Autodesk Inventor part; units mm, degrees
ref_plane "YZ Plane" through (0, 0, 0) normal (1, 0, 0) x (0, 1, 0)
ref_plane "XZ Plane" through (0, 0, 0) normal (0, 1, 0) x (-1, 0, 0)
ref_plane "XY Plane" through (0, 0, 0) normal (0, 0, 1) x (1, 0, 0)
ref_plane "РабПлоскость1" through (-185.8888, -38.5334, 331.0061) normal (0.9999756, 0.0023998, -0.0065586) x (-0.0066118, 0.0228778, -0.9997164)
sketch "Эскиз9" plane through (-185.8888, -38.5334, 331.0061) normal (0.9999756, 0.0023998, -0.0065586) x (-0.0066118, 0.0228778, -0.9997164)
  circle A0 centre (-0.0036, 0) radius 3.25
  line L0 (7.5744, -20.841) -> (-21.2183, 6.4584)
  line L1 (-21.2183, 6.4584) -> (-7.5816, 20.841)
  line L2 (-7.5816, 20.841) -> (21.2112, -6.4584)
  line L3 (21.2112, -6.4584) -> (7.5744, -20.841)
  line L4 (7.5744, -20.841) -> (-7.5816, 20.841) construction
  line L5 (-21.2183, 6.4584) -> (21.2112, -6.4584) construction
  line L6 (9.6794, 4.4753) -> (-3.9573, -9.9074)
  point P0 (330.5647, 30.5274)
extrude "Выдавливание4" add sketch "Эскиз9" along normal blind 6 contours L0 L1 L2 L6
fillet "Сопряжение2" radius 2 8 edges at (-182.8404, -48.5216, 334.7158) (-179.8019, -40.5311, 343.5115) (-185.8017, -40.5455, 343.5509) (-182.963, -33.8307, 321.4122) (-179.9244, -25.8402, 330.2079) (-185.9242, -25.8546, 330.2473) (-185.9016, -41.1833, 328.0837) (-179.9018, -41.1689, 328.0443)
sketch "Эскиз11" plane through (-185.7754, -31.0798, 351.0238) normal (0.0032506, 0.6712535, 0.7412207) x (0.9999756, 0.0023998, -0.0065586)
  line L0 (0, 17.8197) -> (6, -2)
  line L1 (6, 17.8197) -> (0, -2)
  line L2 (2.4, 11.0099) -> (3.6, 11.0099)
  line L3 (3.6, 11.0099) -> (3.6, 4.8099)
  line L4 (3.6, 4.8099) -> (2.4, 4.8099)
  line L5 (2.4, 4.8099) -> (2.4, 11.0099)
  line L6 (2.4, 11.0099) -> (3.6, 4.8099) construction
  line L7 (3.6, 11.0099) -> (2.4, 4.8099) construction
  point P0 (188.1477, 257.5062)
  point P1 (3, 7.9099)
  dimension "d31" = 1.2
  dimension "d32" = 6.2
extrude "Выдавливание6" cut sketch "Эскиз11" against normal blind 6
sketch "Эскиз12" plane through (-179.889, -38.519, 330.9668) normal (0.9999756, 0.0023998, -0.0065586) x (-0.0066118, 0.0228778, -0.9997164)
  line L0 (-16.5329, 11.4001) -> (-12.267, 15.8993)
  line L1 (-16.5329, 11.4001) -> (-12.1788, 7.2719)
  line L2 (-12.1788, 7.2719) -> (-7.913, 11.7711)
  line L3 (-12.267, 15.8993) -> (-7.913, 11.7711)
  line L4 (-12.1788, 7.2719) -> (-12.267, 15.8993)
  line L5 (-16.5329, 11.4001) -> (-7.913, 11.7711)
  circle A0 centre (-12.2229, 11.5856) radius 1.5
  point P0 (330.5647, 30.5274)
  dimension "d35" = 3
extrude "Выдавливание7" cut sketch "Эскиз12" against normal blind 6 contours A0 L4 L5 | L5 L4 A0 | A0 L5 L4 | L4 L5 A0
properties part number "хвост"
Can you work these out from the model? Positions are in its coordinate system, mm. Coordinates: 2 decimals unless noted, no trailing zeros. Return JSON: item names as keys, results as strings. Group by question number.
Item 1: Thinking about a two-plate mould opening in Z: for faces 1 (the cylindrical face through (-182.93, -35.37, 331.77)), 2 (the cylindrical face through (-180.74, -40.84, 328.25)), 3 (the cylindrical face through (-181.03, -27.76, 342.06)), 4 (the cylindrical face through (-185.201, -39.552, 343.792)), which applies, released by +Z, released by -Z, zero draft, split by the parting line, or undercut?
Item 2: Imagine slicing it at A-A (z = 344.5). Give the number of separate pieces and of enclosed holes in the cut face, and give its area (3 significant figures).
Item 3: I'm going to push flat-ended pins straight in: pin 1 Ø10 at (y, z) = (-41, 333.5) entering from -X; pin 2 Ø2 at (x, y) = (-180.5, -33.5) entering from -Z; pin 3 Ø10 at (y, z) = (-44.5, 343) entering from +X; pin 4 Ø2 at (x, y) = (-182.5, -34) entering from -Z. Where does each tip first touch, or does it pass through?
Item 4: If I drill on L1, parallel to X at y = -34.25, z = 324.5; L2, parallel to Y at x = -180.5, z = 333; L3, parallel to Z at x = -183, y = -40, over which ranges is the centre line in solid material (lowest first)? Write a range as from..to.
Verdict:
{
 "1": {"face 1": "undercut", "face 2": "released by -Z", "face 3": "undercut", "face 4": "released by +Z"},
 "2": {"separate pieces": "3", "enclosed holes": "0", "area": "73.9 mm^2"},
 "3": {"pin 1": "stops at x = -185.88", "pin 2": "stops at z = 322.3", "pin 3": "stops at x = -179.82", "pin 4": "stops at z = 322.23"},
 "4": {"L1": "x = -185.94..-179.94", "L2": "y = -45.85..-41.06, -35.98..-24.1", "L3": "z = 327..328.09, 333.89..344.13"}
}
